Autodesk Inventor part; units mm, degrees
ref_plane "YZ Plane" through (0, 0, 0) normal (1, 0, 0) x (0, 1, 0)
ref_plane "XZ Plane" through (0, 0, 0) normal (0, 1, 0) x (-1, 0, 0)
ref_plane "XY Plane" through (0, 0, 0) normal (0, 0, 1) x (1, 0, 0)
sketch "Sketch1" plane through (0, 0, 0) normal (0, 1, 0) x (-1, 0, 0)
  line L0 (7, 12.25) -> (-7, 12.25)
  line L1 (-7, 12.25) -> (-7, -12.25)
  line L2 (-7, -12.25) -> (7, -12.25)
  line L3 (7, -12.25) -> (7, 12.25)
  line L4 (7, 0) -> (-7, 0) construction
  point P0 (0, 0)
  point P1 (0, 0)
  dimension "d0" = 14
  dimension "d1" = 24.5
extrude "Extrusion1" add sketch "Sketch1" along normal blind 13.88
fillet "Fillet1" radius 0.5 12 edges at (7, 6.94, 12.25) (-7, 6.94, 12.25) (-7, 6.94, -12.25) (7, 6.94, -12.25) (7, 13.88, 0) (0, 13.88, -12.25) (-7, 13.88, 0) (0, 13.88, 12.25) (0, 0, 12.25) (7, 0, 0) (0, 0, -12.25) (-7, 0, 0)
sketch "Sketch2" plane through (0, 13.88, 0) normal (0, 1, 0) x (1, 0, 0)
  arc A0 (1, -5.8146) -> (-1, -5.8146) centre (0, 0) ccw
  circle A1 centre (0, 0) radius 3.94
  line L0 (1, -5.8146) -> (1, -5.0646)
  line L1 (1, -5.0646) -> (-1, -5.0646)
  line L2 (-1, -5.0646) -> (-1, -5.8146)
  line L3 (0, 0) -> (0, -5.0646) construction
  dimension "d5" = 11.8
  dimension "d8" = 7.88
  dimension "d9" = 0.75
  dimension "d10" = 2
extrude "Extrusion3" add sketch "Sketch2" along normal blind 11.15
chamfer "Chamfer1" distance 0.5 angle 45 1 edges at (0, 25.03, -5.9)
thread "Thread1"
properties part number "Toggle_Base" material "PC/ABS Plastic"
CAD build for the part. Positions are in the model's coordinates, mm. A direction names the side the tool comes from. Coordinates: 2 decimals unless noted, no trailing zeros. Loops run counter-clockwise (first coordinate to the right, second up) from the corner with the lowest first, then second, coordinate; pieces in that order, holes last. Notation, with made-up numbers: (-20.75, 52) - (21.25, 52) arc R18 ccw to (21.25, 83) - close; hole circle Ø4 at (85.25, -30.75). An arc over 180 degrees is marked (long way). Write item = value, one per line. Start each with the question number.
Q1. Which spindle directions (+Z, -Z, +X, -X, +Y, -Y) get a long thin tool onto all of the face, cutting with end or side? Do faces 1 (the flat face through (0, 19, 5.065)), 2 (the flat face through (1, 25.03, -4)), 3 (the flat face through (0.1, 13.88, 5.4)). Say none if no direction does.
Q2. Cut at D-D, the plane z = -9.5. List the corners of the cut face in (x, y).
Q3. Cut at B-B, the plane y = 19.5. List the corners of the cut face in (x, z), then the cut area to 3 significant figures.
Q4. Flat gauge pin, fed straight in: pin 1 Ø2.5 at (x, z) = (-1, -1) entering from +Y. Where does the tip first touch, or does it go through?
Q5. Drill centre lines: L1, parallel to Z at x = 0, y = 22.5; L2, parallel to Y at x = 1.5, z = -9.5; L3, parallel to X at y = 18, z = 0. Where is each one in solid material? Low to high.
Q6. Cut at A-A, the plane x = 0. List the corners of the cut face in (y, z), then the cut area to 3 significant figures.
Q7. Cut at C-C, the plane z = 0. List the corners of the cut face in (x, y).
Q8. Pull direction X, two halves, no side cores. Call faces 4 (the flat face through (0, 0, 0)), 5 (the flat face through (-7, 7, 0)), 6 (the cylindrical face through (-0.854, 19.377, -3.846)), 7 (the flat face through (0, 13.88, 0)): pulls with the +X half, pulls with the -X half, needs draft (parallel to the pull), parting line crosses it, or undercut.
Computed:
q1.face_1 = +Z, +Y
q1.face_2 = +Z, -Z, +X, -X, +Y
q1.face_3 = +Y
q2.outline = (-7, 0.5) arc R0.5 ccw to (-6.5, 0) - (6.5, 0) arc R0.5 ccw to (7, 0.5) - (7, 13.38) arc R0.5 ccw to (6.5, 13.88) - (-6.5, 13.88) arc R0.5 ccw to (-7, 13.38) - close
q3.outline = (-1, 5.06) - (-1, 5.81) arc R5.9 ccw (long way) to (1, 5.81) - (1, 5.06) - close; hole circle Ø7.88 at (0, 0)
q3.area = 59.0 mm²
q4.pin_1 = 13.88
q5.L1 = -5.9 to -3.94, 3.94 to 5.06
q5.L2 = 0 to 13.88
q5.L3 = -5.9 to -3.94, 3.94 to 5.9
q6.outline = (0, -11.75) arc R0.5 ccw to (0.5, -12.25) - (13.38, -12.25) arc R0.5 ccw to (13.88, -11.75) - (13.88, -5.9) - (24.53, -5.9) - (25.03, -5.4) - (25.03, -3.94) - (13.88, -3.94) - (13.88, 3.94) - (25.03, 3.94) - (25.03, 5.06) - (13.88, 5.06) - (13.88, 11.75) arc R0.5 ccw to (13.38, 12.25) - (0.5, 12.25) arc R0.5 ccw to (0, 11.75) - close
q6.area = 374 mm²
q7.outline = (-7, 0.5) arc R0.5 ccw to (-6.5, 0) - (6.5, 0) arc R0.5 ccw to (7, 0.5) - (7, 13.38) arc R0.5 ccw to (6.5, 13.88) - (5.9, 13.88) - (5.9, 24.53) - (5.4, 25.03) - (3.94, 25.03) - (3.94, 13.88) - (-3.94, 13.88) - (-3.94, 25.03) - (-5.4, 25.03) - (-5.9, 24.53) - (-5.9, 13.88) - (-6.5, 13.88) arc R0.5 ccw to (-7, 13.38) - close
q8.face_4 = needs draft
q8.face_5 = pulls with the -X half
q8.face_6 = undercut
q8.face_7 = undercut
